Input: dimensioned drawing with shaded views. Units: mm. Origin: part minimum x, y, z. A direction names the side the tool comes from. Round coordinates to 2 decimals unless told otherwise and drop trailing zeros. Loops run counter-clockwise (first coordinate to the right, second up) from the corner with the lowest first, then second, coordinate; pieces in that order, holes last.
1) Access query for the marked faces 1, 2, 3, 4 and 5. Directions: +Z, -Z, +X, -X, +Y, -Y. A direction counts if a zero-diameter tool reaches every point of the face in a straight line with its end or side. Return the directions, or none.
2) Section A-A, the plane x = 17.75. Return loops of the section in (y, z), and give its area (3 significant figures).
3) Section D-D, the plane x = 10.75. Return loops of the section in (y, z), and give its area (3 significant figures).
4) First-contact query: pin 1 (0.6 mm diameter, centred on y = 12.5, z = 4, fed in from +X); pin 2 (1.5 mm diameter, centred on x = 15.5, z = 3, fed in from +Y); pin 3 (2.5 mm diameter, centred on x = 17.5, z = 5.5, fed in from +Y); pin 4 (5.5 mm diameter, centred on x = 13, y = 2, fed in from -Z). Flat tips, straight axial feed; report the tip coordinate or a pass-through.
5) Section C-C, the plane y = 7.5. Return loops of the section in (x, z), and give its area (3 significant figures).
6) Ray query, line 1 along Z through (x, y) = (2.5, 11.25); line 2 along Y through (x, z) = (17.25, 6.5); line 3 along Z through (x, y) = (15.75, 16.5). Return the intervals inside material, ascending.
7) Section B-B, the plane z = 3. Return loops of the section in (x, y), and give its area (3 significant figures).
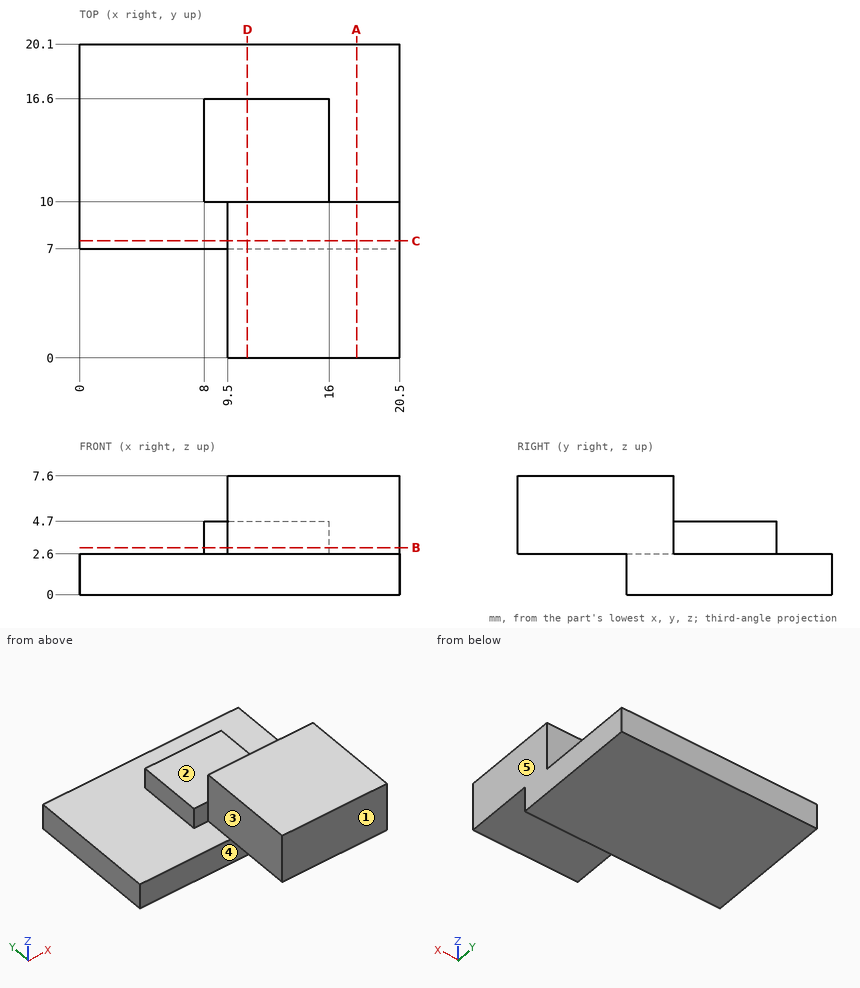
Final values:
1. face 1: +Z, -Z, +X, -X, -Y
1. face 2: +Z, +X, -X, +Y
1. face 3: +Z, -X, -Y
1. face 4: -Z, +X, -X, -Y
1. face 5: +Z, -Z, +X, +Y, -Y
2. outline: (0, 2.6) - (7, 2.6) - (7, 0) - (20.1, 0) - (20.1, 2.6) - (10, 2.6) - (10, 7.6) - (0, 7.6) - close
2. area: 84.1 mm2
3. outline: (0, 2.6) - (7, 2.6) - (7, 0) - (20.1, 0) - (20.1, 2.6) - (16.6, 2.6) - (16.6, 4.7) - (10, 4.7) - (10, 7.6) - (0, 7.6) - close
3. area: 97.9 mm2
4. pin 1: stops at x = 16
4. pin 2: stops at y = 20.1
4. pin 3: stops at y = 10
4. pin 4: stops at z = 2.6
5. outline: (0, 0) - (20.5, 0) - (20.5, 7.6) - (9.5, 7.6) - (9.5, 2.6) - (0, 2.6) - close
5. area: 108 mm2
6. line 1: z = 0 to 2.6
6. line 2: y = 0 to 10
6. line 3: z = 0 to 4.7
7. outline: (8, 10) - (9.5, 10) - (9.5, 0) - (20.5, 0) - (20.5, 10) - (16, 10) - (16, 16.6) - (8, 16.6) - close
7. area: 163 mm2
